Here's how the part is built. I have some questions about the finished solid (model axes, mm). Coordinates: 2 decimals unless noted, no trailing zeros. Write each loop counter-clockwise with the first axis right and the second up, starting at its lowest first coordinate (ties: lowest second). Pieces come first, ordered by that corner, then holes.
Item 1: Please list where these lines run through material, in increasing order: line 1 (Z direction, x = 2.2, y = 12.7) (3 decimals); line 2 (Z direction, x = 2.1, y = 44.45) (3 decimals); line 3 (Y direction, x = 1.7, z = 103).
Item 2: I'm going to push flat-ended pins straight in: P1, Ø5.5, axis at y = 12.7, z = 50.8, coming from the -X side; P2, Ø1.5, axis at x = 2, y = 28.5, coming from the +Z side. Where does each tip first touch, or does it pass through?
Item 3: I want a section at B-B (y = 12.7). Please give me the cut outline in (x, z) (3 decimals), and give its area (3 significant figures).
Item 4: I want a section at A-A (z = 12.7). Please give me the cut outline in (x, y) (3 decimals), and give its area (3 significant figures).
Item 5: I want a section at C-C (x = 0.85). Please give me the cut outline in (y, z) (3 decimals), and give its area (3 significant figures).
Item 6: I want a section at D-D (y = 44.45). Please give me the cut outline in (x, z) (3 decimals).
Item 7: If we mould it in two halves opening along Z, with no side actions, what happens to faces 1 (the face through (2, 39, 0)), 2 (the face through (3.175, 21, 43)), 3 (the face through (1.57, 14.63, 104.12))? For each: pulls with the +Z half, pulls with the -Z half, needs draft (parallel to the pull), parting line crosses it, or undercut.
Autodesk Inventor part; units mm, degrees
ref_plane "YZ Plane" through (0, 0, 0) normal (1, 0, 0) x (0, 1, 0)
ref_plane "XZ Plane" through (0, 0, 0) normal (0, 1, 0) x (-1, 0, 0)
ref_plane "XY Plane" through (0, 0, 0) normal (0, 0, 1) x (1, 0, 0)
sketch "Sketch1" plane through (0, 0, 0) normal (1, 0, 0) x (0, 1, 0)
  line L0 (0, 0) -> (0, 152.4)
  line L1 (0, 152.4) -> (76.2, 0)
  line L2 (76.2, 0) -> (0, 0)
  dimension "d0" = 152.4
  dimension "d1" = 76.2
extrude "Extrusion1" add sketch "Sketch1" along normal blind 3.175
sketch "Sketch2" plane through (3.175, 0, 0) normal (1, 0, 0) x (0, 0, -1)
  line L0 (-152.4, 0) -> (0, 0)
  line L1 (0, 0) -> (0, 76.2)
  point P0 (-12.7, 44.45)
  point P1 (-12.7, 19.05)
  dimension "d4" = 12.7
  dimension "d5" = 12.7
  dimension "d6" = 19.05
  dimension "d7" = 25.4
hole "Hole2" at (3.175, 44.45, 12.7) at (3.175, 19.05, 12.7) direction (-1, 0, 0) diameter 6.35 end through all
sketch "Sketch4" plane through (3.175, 0, 0) normal (1, 0, 0) x (0, 0, -1)
  line L0 (-152.4, 0) -> (0, 0)
  line L1 (0, 0) -> (0, 76.2)
  point P0 (-101.6, 12.7)
  point P1 (-50.8, 12.7)
  dimension "d25" = 12.7
  dimension "d26" = 12.7
  dimension "d27" = 50.8
  dimension "d28" = 50.8
hole "Hole3" at (3.175, 12.7, 101.6) at (3.175, 12.7, 50.8) direction (-1, 0, 0) diameter 6.35 end through all
properties part number "Support_Side_Front" material "Aluminum 6061"
Answer:
1. line 1: z = 0 to 47.625, 53.975 to 98.425, 104.775 to 127
1. line 2: z = 0 to 9.525, 15.875 to 63.5
1. line 3: y = 0 to 9.85, 15.55 to 24.7
2. P1: passes through
2. P2: stops at z = 96.9
3. outline: (0, 0) - (3.175, 0) - (3.175, 47.625) - (0, 47.625) - close; (0, 53.975) - (3.175, 53.975) - (3.175, 98.425) - (0, 98.425) - close; (0, 104.775) - (3.175, 104.775) - (3.175, 127) - (0, 127) - close
3. area: 363 mm2
4. outline: (0, 0) - (3.175, 0) - (3.175, 15.875) - (0, 15.875) - close; (0, 22.225) - (3.175, 22.225) - (3.175, 41.275) - (0, 41.275) - close; (0, 47.625) - (3.175, 47.625) - (3.175, 69.85) - (0, 69.85) - close
4. area: 181 mm2
5. outline: (0, 0) - (76.2, 0) - (0, 152.4) - close; hole circle Ø6.35 at (12.7, 50.8); hole circle Ø6.35 at (12.7, 101.6); hole circle Ø6.35 at (19.05, 12.7); hole circle Ø6.35 at (44.45, 12.7)
5. area: 5,680 mm2
6. outline: (0, 0) - (3.175, 0) - (3.175, 9.525) - (0, 9.525) - close; (0, 15.875) - (3.175, 15.875) - (3.175, 63.5) - (0, 63.5) - close
7. face 1: pulls with the -Z half
7. face 2: needs draft
7. face 3: undercut
